Input: part model. Units: mm. Frame: model coordinates. A direction names the side the tool comes from. Give positions to 0.01 mm unless a question says otherwise; leave off trailing zeros. Loops run counter-clockwise (first coordinate to the right, second up) from the corner with the lowest first, then second, coordinate; pieces in that order, holes last. Notation, with made-up numbers: (-6, -37.5) -> (44, -37.5) arc R20 cw to (44, 0.5) -> close; hole circle Ø1 at (-34, 5.5). An arc over 180 degrees is marked (long way). Answer as a JSON object with one key per item and string values.
```python
from build123d import *

# Parameters (mm, degrees)
SKETCH1_R           = 1.650000007
BOSS_EXTRUDE1_DEPTH = 3.5
BOSS_EXTRUDE3_DEPTH = 30
FILLET1_R           = 5
FILLET2_R           = 2
SKETCH4_R           = 9.5
BOSS_EXTRUDE4_DEPTH = 30
FILLET3_R           = 1
REVOLVE1_ANGLE      = 180
SKETCH6_R           = 5
CUT_EXTRUDE1_DEPTH  = 10
SKETCH7_R           = 1.6
CUT_EXTRUDE2_DEPTH  = 10


with BuildPart() as part:
    # Sketch1 → Boss-Extrude1 (new, symmetric)
    with BuildSketch(Plane(origin=(0, 0, 0), x_dir=(1, 0, 0), z_dir=(0, 1, 0))):
        with BuildLine():
            Line((-56.656859897, 90.483506167), (-36.993673105, 86.828497938))
            ThreePointArc((-36.993673105, 86.828497938), (-33.173282872, 84.013663947), (-34.729774781, 79.530807173))
            Line((-34.729774781, 79.530807173), (-58.047969803, 63.522628609))
            ThreePointArc((-58.047969803, 63.522628609), (-61.213536363, 62.923269927), (-63.79414326, 64.852132418))
            ThreePointArc((-63.79414326, 64.852132418), (-64.662572796, 65.817505246), (-65.857598376, 66.32547022))
            Line((-65.857598376, 66.32547022), (-94.996570641, 71.741844715))
            ThreePointArc((-94.996570641, 71.741844715), (-96.92158748, 72.993398991), (-97.397797425, 75.239573968))
            Line((-97.397797425, 75.239573968), (-94.29104043, 91.953282742))
            ThreePointArc((-94.29104043, 91.953282742), (-93.039486154, 93.878299581), (-90.793311177, 94.354509526))
            Line((-90.793311177, 94.354509526), (-61.654338999, 88.938135048))
            ThreePointArc((-61.654338999, 88.938135048), (-60.356600681, 88.982743171), (-59.199275822, 89.571567253))
            ThreePointArc((-59.199275822, 89.571567253), (-58.007370108, 90.248625312), (-56.656859897, 90.483506167))
        make_face()
        with Locations(Location((-56.656859897, 86.483506167, 0), (0, 0, 270))):
            Circle(SKETCH1_R, mode=Mode.SUBTRACT)
        with Locations(Location((-36.993673105, 82.828497938, 0), (0, 0, 270))):
            Circle(SKETCH1_R, mode=Mode.SUBTRACT)
        with Locations(Location((-60.311868127, 66.820319374, 0), (0, 0, 270))):
            Circle(SKETCH1_R, mode=Mode.SUBTRACT)
    extrude(amount=BOSS_EXTRUDE1_DEPTH, both=True)

    # Sketch3 → Boss-Extrude3 (add)
    with BuildSketch(Plane(origin=(0, -3.5, 0), x_dir=(1, 0, 0), z_dir=(0, 1, 0))):
        with BuildLine():
            Line((-69.163805705, 90.334000474), (-90.793311177, 94.354509526))
            ThreePointArc((-90.793311177, 94.354509526), (-93.039486154, 93.878299581), (-94.29104043, 91.953282742))
            Line((-94.29104043, 91.953282742), (-97.397797425, 75.239573968))
            ThreePointArc((-97.397797425, 75.239573968), (-96.92158748, 72.993398991), (-94.996570641, 71.741844715))
            Line((-94.996570641, 71.741844715), (-73.367065169, 67.721335662))
            ThreePointArc((-73.367065169, 67.721335662), (-71.120890192, 68.197545608), (-69.869335915, 70.122562447))
            Line((-69.869335915, 70.122562447), (-66.762578921, 86.836271221))
            ThreePointArc((-66.762578921, 86.836271221), (-67.238788866, 89.082446198), (-69.163805705, 90.334000474))
        make_face()
    extrude(amount=-BOSS_EXTRUDE3_DEPTH)

    # Fillet1
    # the kernel refuses this fillet: 5 mm, written as the material it adds along each edge
    with BuildSketch(Plane(origin=(-72.818813934, -3.5, -70.670813681), x_dir=(0.9358033400655833, 0, -0.35252249392357676), z_dir=(0.35252249392357676, 0, 0.9358033400655833))) as fillet1_piece_1_section:
        with BuildLine():
            CenterArc((3 + FILLET1_R, -FILLET1_R), FILLET1_R, 90, 90)
            Line((3 + FILLET1_R, 0), (3, 0))
            Line((3, 0), (3, -FILLET1_R))
        make_face()
    fillet1_piece_1 = revolve(axis=Axis((-72.818813934, -3.5, -70.670813681), (0, 1, 0)), revolution_arc=328.828315396, mode=Mode.PRIVATE)
    fillet1_piece_1 = split(fillet1_piece_1, bisect_by=Plane(origin=(-73.367065169, -3.5, -67.721335662), z_dir=(0.18275041146570634, 0, -0.9831593396337722)), keep=Keep.TOP, mode=Mode.PRIVATE)
    add(fillet1_piece_1)
    with BuildSketch(Plane(origin=(-69.869335915, -3.5, -70.122562447), x_dir=(0, -1, 0), z_dir=(0.18275041146570747, 0, -0.9831593396337721))) as fillet1_piece_2:
        with BuildLine():
            CenterArc((FILLET1_R, -FILLET1_R), FILLET1_R, 90, 90)
            Line((0, -FILLET1_R), (0, 0))
            Line((0, 0), (FILLET1_R, 0))
        make_face()
    extrude(amount=17)
    with BuildSketch(Plane(origin=(-69.712056939, -3.5, -87.384522455), x_dir=(0.9831593396337688, 0, 0.18275041146572465), z_dir=(-0.18275041146572465, 0, 0.9831593396337688))) as fillet1_piece_3_section:
        with BuildLine():
            CenterArc((3 + FILLET1_R, -FILLET1_R), FILLET1_R, 90, 90)
            Line((3 + FILLET1_R, 0), (3, 0))
            Line((3, 0), (3, -FILLET1_R))
        make_face()
    fillet1_piece_3 = revolve(axis=Axis((-69.712056939, -3.5, -87.384522455), (0, 1, 0)), revolution_arc=328.828315396, mode=Mode.PRIVATE)
    fillet1_piece_3 = split(fillet1_piece_3, bisect_by=Plane(origin=(-69.163805705, -3.5, -90.334000474), z_dir=(-0.1827504114659838, 0, 0.9831593396337207)), keep=Keep.TOP, mode=Mode.PRIVATE)
    add(fillet1_piece_3)

    # Fillet2
    fillet2_edges = [part.edges().sort_by_distance(p)[0] for p in [
        (-71.120890192, -33.5, -68.197545608),
        (-84.181817905, -33.5, -69.731590188),
        (-96.92158748, -33.5, -72.993398991),
        (-95.844418928, -33.5, -83.596428355),
        (-93.039486154, -33.5, -93.878299581),
        (-79.978558441, -33.5, -92.344255),
        (-67.238788866, -33.5, -89.082446198),
        (-68.315957418, -33.5, -78.479416834),
    ]]
    fillet(fillet2_edges, radius=FILLET2_R)

    # Sketch4 → Boss-Extrude4 (add)
    with BuildSketch(Plane(origin=(0, -33.5, 0), x_dir=(-1, 0, 0), z_dir=(0, -1, 0))):
        with Locations(Location((82.080188173, 81.037922594, 0), (0, 0, 280.530004657))):
            Circle(SKETCH4_R)
    extrude(amount=BOSS_EXTRUDE4_DEPTH)

    # Fillet3
    fillet3_edges = [part.edges().sort_by_distance(p)[0] for p in [
        (-72.740174433, -33.5, -79.301793759),
        (-91.420201913, -33.5, -82.77405143),
    ]]
    fillet(fillet3_edges, radius=FILLET3_R)

    # Sketch5 → Revolve1 (revolve)
    with BuildSketch(Plane(origin=(0, -63.5, 0), x_dir=(-1, 0, 0), z_dir=(0, -1, 0))):
        with BuildLine():
            Line((82.080188173, 90.537922594), (82.080188173, 71.537922594))
            ThreePointArc((82.080188173, 71.537922594), (91.580188173, 81.037922594), (82.080188173, 90.537922594))
        make_face()
    revolve(axis=Axis((-82.080188173, -63.5, -90.537922594), (0, 0, 1)), revolution_arc=REVOLVE1_ANGLE)

    # Sketch6 → Cut-Extrude1 (cut)
    with BuildSketch(Plane(origin=(0, 3.5, 0), x_dir=(1, 0, 0), z_dir=(0, 1, 0))):
        with Locations((-44.086083588, 88.146840634)):
            Circle(SKETCH6_R)
    extrude(amount=-CUT_EXTRUDE1_DEPTH, mode=Mode.SUBTRACT)

    # Sketch7 → Cut-Extrude2 (cut)
    with BuildSketch(Plane(origin=(0, 3.5, 0), x_dir=(1, 0, 0), z_dir=(0, 1, 0))):
        with Locations(Location((-88.848960421, 88.398881924, 0), (0, 0, 270))):
            Circle(SKETCH7_R)
        with Locations(Location((-91.041965359, 76.600969848, 0), (0, 0, 270))):
            Circle(SKETCH7_R)
        with Locations(Location((-75.084729666, 85.840376163, 0), (0, 0, 270))):
            Circle(SKETCH7_R)
        with Locations(Location((-77.277734604, 74.042464088, 0), (0, 0, 270))):
            Circle(SKETCH7_R)
    extrude(amount=-CUT_EXTRUDE2_DEPTH, mode=Mode.SUBTRACT)


solid = part.part
```
Q1. Access query for faces 4 (the flat face through (-93, -33.5, -83)), 5 (the flat face through (-77, -6.5, -74)), 6 (the cylindrical face through (-58.03, 0.05, -90.24)). Directions: +Z, -Z, +X, -X, +Y, -Y. A direction counts if a zero-diameter tool reaches every point of the face in a straight line with its end or side. Return the directions, or none.
Evaluation:
{"face 4": "-X, -Y", "face 5": "+Y", "face 6": "-Z, +Y, -Y"}
Q2. Section B-B, the plane x = -45. Return the cut outline in (y, z).
Evaluation:
{"outline": "(-3.5, -83.23) -> (3.5, -83.23) -> (3.5, -72.48) -> (-3.5, -72.48) -> close"}
Q3. Section A-A, the plane y = -49. Return the cut outline in (x, z), then the cut area to 3 significant figures.
Evaluation:
{"outline": "circle Ø19 at (-82.08, -81.04)", "area": "284 mm2"}
Q4. Pin query (flat end, axial travel): pin 1 (5.5 mm diameter, centred on x = -92, z = -86.5, fed in from -Y); pin 2 (1 mm diameter, centred on x = -89, z = -88, fed in from +Y); pin 3 (3 mm diameter, centred on x = -88.85, z = -88.4, fed in from -Y); pin 4 (2 mm diameter, centred on x = -60.31, z = -66.82, fed in from -Y). Return the tip coordinate at first contact, or that it passes through.
Evaluation:
{"pin 1": "stops at y = -67.59", "pin 2": "stops at y = -6.5", "pin 3": "stops at y = -67.74", "pin 4": "passes through"}
Q5. Ray query, line 1 along X through (y, z) = (-6, -75.5); line 2 along X through (y, z) = (-48, -80.5); line 3 along Z through (x, y) = (-81.5, -52.5). Return the intervals inside material, ascending.
Evaluation:
{"line 1": "x = -97.35 to -92.2, -89.88 to -77.94, -76.62 to -68.19", "line 2": "x = -91.56 to -72.6", "line 3": "z = -90.52 to -71.56"}
Q6. Draft query along X for faces 1 (the flat face through (-89, -6.5, -88)), 2 (the cylindrical face through (-33.2, 0, -84.1)), 3 (the cylindrical face through (-80.107, -48.673, -71.745)). Return one class per face: +X half, -X half, draft (parallel to the pull), parting line (faces both ways), or undercut.
Evaluation:
{"face 1": "undercut", "face 2": "+X half", "face 3": "parting line"}
